For this review, take the finished solid that the model builds, in its own axes (mm). Face numbers are marked on the shaded views. A direction names the side the tool comes from. Coordinates: 2 decimals unless noted, no trailing zeros. Write each loop counter-clockwise with the first axis right and the second up, starting at its lowest first coordinate (ties: lowest second). Pieces come first, ordered by that corner, then holes. Notation, with made-up numbers: (60.5, 21.25) - (80.5, 21.25) arc R19 ccw to (80.5, 44.25) - close; hole circle Ø4 at (89, -2.75). An arc over 180 degrees is marked (long way). Use one line per item in the form item = value. Start each with the question number.
1) Mouldability with a two-part tool opening along Y and no side actions: class the marked faces 1 and 2 as pulls with the +Y half, pulls with the -Y half, needs draft (parallel to the pull), parting line crosses it, or undercut.
2) We need section D-D (y = -20). Give the boundary of the cut face in (x, z), plus the area to 3 significant figures.
3) Tool access review of the marked faces 3, 4 and 5: name each direction out of +Z, -Z, +X, -X, +Y, -Y from which nothing blocks a thin tool from reaching the whole face with its end or side.
4) We need section A-A (x = 0). Give the boundary of the cut face in (y, z).
5) For L1, parallel to Y at x = 0, z = 3.1; L2, parallel to X at y = -5, z = -8.5; L3, parallel to Y at x = -20.5, z = -2.75, list the stretches that pass through material, from the lowest coordinate up. Write a range as from..to.
6) We need section C-C (z = 11). Give the boundary of the cut face in (x, y), plus the area to 3 significant figures.
7) We need section B-B (x = 26.5). Give the boundary of the cut face in (y, z).
8) Insertion check: P1, Ø1.1, axis at x = -24, z = 5, coming from the +Y side; P2, Ø4, axis at x = -20, z = -5, coming from the +Y side; P3, Ø2, axis at y = 15.5, z = 4, coming from the +X side. Each pin has a flat end and moves straight along its axis. Give the tip position at first contact, or say it passes through.
```python
from build123d import *
from build123d.topology import SkipClean

# Parameters (mm, degrees)
SKETCH1_R           = 29.95
BOSS_EXTRUDE1_DEPTH = 12.7
SKETCH3_R           = 12
CUT_EXTRUDE2_DEPTH  = 45.218717756
SKETCH4_R           = 12
BOSS_EXTRUDE2_DEPTH = 2.2225
SKETCH5_R           = 8.95
CUT_EXTRUDE3_DEPTH  = 43.852874193
BOSS_EXTRUDE6_START = 13.5
SKETCH11_R          = 29.95
SKETCH11_R_2        = 12
BOSS_EXTRUDE6_DEPTH = 13.5
SKETCH12_R          = 4.05
CUT_EXTRUDE4_DEPTH  = 14.5
BOSS_EXTRUDE7_START = 4
SKETCH14_R          = 4.05
BOSS_EXTRUDE7_DEPTH = 4
SKETCH16_R          = 3
CUT_EXTRUDE5_DEPTH  = 4
CUT_EXTRUDE6_DEPTH  = 8


with BuildPart() as part:
    # Sketch1 → Boss-Extrude1 (new body)
    with BuildSketch(Plane.XY):
        Circle(SKETCH1_R)
    extrude(amount=BOSS_EXTRUDE1_DEPTH)

    # Sketch3 → Cut-Extrude2 (cut, through all)
    with BuildSketch(Plane(origin=(0, 0, 0), x_dir=(-1, 0, 0), z_dir=(0, 0, -1))):
        Circle(SKETCH3_R)
    extrude(amount=-CUT_EXTRUDE2_DEPTH, mode=Mode.SUBTRACT)

    # Sketch4 → Boss-Extrude2 (add)
    with BuildSketch(Plane(origin=(0, 0, 3.96875), x_dir=(-1, 0, 0), z_dir=(0, 0, -1))):
        Circle(SKETCH4_R)
    extrude(amount=-BOSS_EXTRUDE2_DEPTH)

    # Sketch5 → Cut-Extrude3 (cut, through all)
    with BuildSketch(Plane.XY.offset(6.19125)):
        Circle(SKETCH5_R)
    extrude(amount=-CUT_EXTRUDE3_DEPTH, mode=Mode.SUBTRACT)

    # Sketch11 → Boss-Extrude6 (add)
    with BuildSketch(Plane(origin=(0, 0, 0), x_dir=(-1, 0, 0), z_dir=(0, 0, -1)).offset(BOSS_EXTRUDE6_START)):
        Circle(SKETCH11_R)
        Circle(SKETCH11_R_2, mode=Mode.SUBTRACT)
    extrude(amount=-BOSS_EXTRUDE6_DEPTH)

    # Sketch12 → Cut-Extrude4 (cut)
    with BuildSketch(Plane(origin=(-29.95, 0, 6.19125), x_dir=(0, 0, 1), z_dir=(-1, 0, 0))):
        with Locations((-6.59125, 0)):
            Circle(SKETCH12_R)
    cut_extrude4 = extrude(amount=-CUT_EXTRUDE4_DEPTH, mode=Mode.SUBTRACT)

    # Sketch14 → Boss-Extrude7 (add)
    with BuildSketch(Plane(origin=(-16.95, 0, 6.19125), x_dir=(0, 0, 1), z_dir=(-1, 0, 0)).offset(BOSS_EXTRUDE7_START)):
        with Locations((-6.59125, 0)):
            Circle(SKETCH14_R)
    boss_extrude7 = extrude(amount=-BOSS_EXTRUDE7_DEPTH)

    # Sketch16 → Cut-Extrude5 (cut)
    with BuildSketch(Plane.ZY.offset(20.95)):
        with Locations((-0.4, 0)):
            Circle(SKETCH16_R)
    cut_extrude5 = extrude(amount=-CUT_EXTRUDE5_DEPTH, mode=Mode.SUBTRACT)

    # Sketch17 → Cut-Extrude6 (cut)
    with BuildSketch(Plane(origin=(-29.95, 0, 6.19125), x_dir=(0, 0, 1), z_dir=(-1, 0, 0))):
        with BuildLine():
            Line((0.530468331, 2), (-3.069531669, 2))
            ThreePointArc((-3.069531669, 2), (-2.54125, 0), (-3.069531669, -2))
            Line((-3.069531669, -2), (0.530468331, -2))
            ThreePointArc((0.530468331, -2), (1.237575112, -1.707106781), (1.530468331, -1))
            Line((1.530468331, -1), (1.530468331, 1))
            ThreePointArc((1.530468331, 1), (1.237575112, 1.707106781), (0.530468331, 2))
        make_face()
        with BuildLine():
            Line((-14.712968331, -2), (-10.112968331, -2))
            ThreePointArc((-10.112968331, -2), (-10.64125, 0), (-10.112968331, 2))
            Line((-10.112968331, 2), (-14.712968331, 2))
            Line((-14.712968331, 2), (-14.712968331, -2))
        make_face()
    cut_extrude6 = extrude(amount=-CUT_EXTRUDE6_DEPTH, mode=Mode.SUBTRACT)

    # Mirror1: Cut-Extrude4, Boss-Extrude7, Cut-Extrude5, Cut-Extrude6 across plane
    with SkipClean():  # the faces are left unmerged after this step: merging them gives an invalid solid
        add(cut_extrude4.mirror(Plane.ZY), mode=Mode.SUBTRACT)
        add(boss_extrude7.mirror(Plane.ZY))
        add(cut_extrude5.mirror(Plane.ZY), mode=Mode.SUBTRACT)
        add(cut_extrude6.mirror(Plane.ZY), mode=Mode.SUBTRACT)


solid = part.part
```
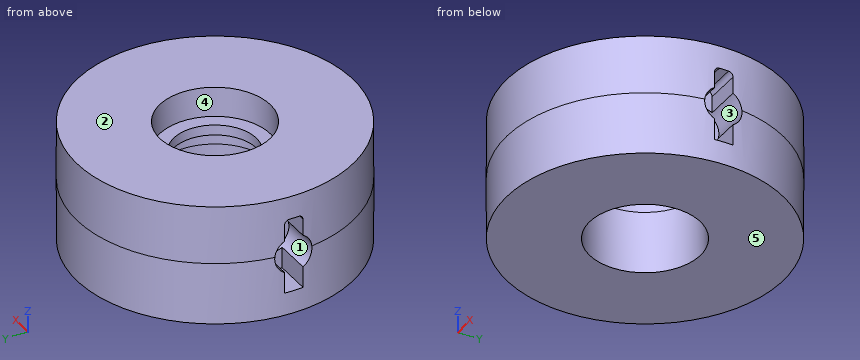
Determined:
q1.face_1 = undercut
q1.face_2 = needs draft
q2.outline = (-22.29, -13.5) - (22.29, -13.5) - (22.29, 12.7) - (-22.29, 12.7) - close
q2.area = 1,170 mm²
q3.face_3 = +X
q3.face_4 = +Z
q3.face_5 = -Z, +X, -X, +Y, -Y
q4.outline = (-29.95, -13.5) - (-12, -13.5) - (-12, 3.97) - (-8.95, 3.97) - (-8.95, 6.19) - (-12, 6.19) - (-12, 12.7) - (-29.95, 12.7) - close; (8.95, 3.97) - (12, 3.97) - (12, -13.5) - (29.95, -13.5) - (29.95, 12.7) - (12, 12.7) - (12, 6.19) - (8.95, 6.19) - close
q5.L1 = -29.95..-12, 12..29.95
q5.L2 = -29.53..-10.91, 10.91..29.53
q5.L3 = -21.83..-1.86, 1.86..21.83
q6.outline = circle Ø59.9 at (0, 0); hole circle Ø24 at (0, 0)
q6.area = 2,370 mm²
q7.outline = (-13.96, -13.5) - (13.96, -13.5) - (13.96, 12.7) - (-13.96, 12.7) - close; hole (-2, -8.52) - (2, -8.52) - (2, -3.92) arc R4.05 ccw to (2, 3.12) - (2, 6.72) arc R1 ccw to (1, 7.72) - (-1, 7.72) arc R1 ccw to (-2, 6.72) - (-2, 3.12) arc R4.05 ccw to (-2, -3.92) - close
q8.P1 = 18.63
q8.P2 = 23.94
q8.P3 = 26.21
